```python
from build123d import *

# Parameters (mm, degrees)
BOSS_EXTRU_1_DEPTH      = 10
COQUE1_T                = 2.5
CONG_1_R                = 2
ESQUISSE3_R             = 3
ESQUISSE3_R_2           = 1.5
BOSS_EXTRU_2_DEPTH      = 9.43
ESQUISSE4_W             = 9.967172774
ESQUISSE4_H             = 2.559848265
ENL_V_MAT_EXTRU_2_DEPTH = 1
CONG_4_R                = 1
ESQUISSE5_R             = 1.7
ESQUISSE5_R_2           = 1.728785314
ESQUISSE5_R_3           = 14.25
ESQUISSE5_R_4           = 14.15
ENL_V_MAT_EXTRU_3_DEPTH = 10
ESQUISSE6_R             = 1.5
ENL_V_MAT_EXTRU_4_DEPTH = 10


# Some blends are built 0.0001 mm under size
with BuildPart() as part:
    # Esquisse1 → Boss.-Extru.1 (new body)
    with BuildSketch(Plane.XY):
        with BuildLine():
            Line((-34.96, -64), (34.96, -64))
            ThreePointArc((34.96, -64), (36.756051224, -63.256051224), (37.5, -61.46))
            Line((37.5, -61.46), (37.5, 61.46))
            ThreePointArc((37.5, 61.46), (36.756051224, 63.256051224), (34.96, 64))
            Line((34.96, 64), (-34.96, 64))
            ThreePointArc((-34.96, 64), (-36.756051224, 63.256051224), (-37.5, 61.46))
            Line((-37.5, 61.46), (-37.5, -61.46))
            ThreePointArc((-37.5, -61.46), (-36.756051224, -63.256051224), (-34.96, -64))
        make_face()
    extrude(amount=BOSS_EXTRU_1_DEPTH)

    # Coque1
    coque1_openings = [part.faces().sort_by_distance(p)[0] for p in [
        (0, 0, 10),
    ]]
    offset(amount=COQUE1_T, openings=coque1_openings, kind=Kind.INTERSECTION)

    # Congé1
    # the kernel refuses this fillet: 2 mm, written as the material it takes off along each edge
    with BuildSketch(Plane(origin=(34.96, 66.5, -2.5), x_dir=(0, 0, 1), z_dir=(-1, 0, 0)), Plane(origin=(-34.96, -66.5, -2.5), x_dir=(0, 0, 1), z_dir=(1, 0, 0))) as cong_1_piece_1:
        with BuildLine():
            CenterArc((CONG_1_R, -CONG_1_R), CONG_1_R, 90, 90)
            Line((0, -CONG_1_R), (0, 0))
            Line((0, 0), (CONG_1_R, 0))
        make_face()
    extrude(amount=69.92, mode=Mode.SUBTRACT)
    with BuildSketch(Plane(origin=(34.96, 61.46, -2.5), x_dir=(0, 1, 0), z_dir=(-1, 0, 0))) as cong_1_piece_2:
        with BuildLine():
            CenterArc((5.04 - CONG_1_R, -CONG_1_R), CONG_1_R, 0, 90)
            Line((5.04 - CONG_1_R, 0), (5.04, 0))
            Line((5.04, 0), (5.04, -CONG_1_R))
        make_face()
    revolve(axis=Axis((34.96, 61.46, -2.5), (0, 0, -1)), revolution_arc=90, mode=Mode.SUBTRACT)
    with BuildSketch(Plane(origin=(40, -61.46, -2.5), x_dir=(0, 0, 1), z_dir=(0, 1, 0)), Plane(origin=(-40, 61.46, -2.5), x_dir=(0, 0, 1), z_dir=(0, -1, 0))) as cong_1_piece_3:
        with BuildLine():
            CenterArc((CONG_1_R, -CONG_1_R), CONG_1_R, 90, 90)
            Line((0, -CONG_1_R), (0, 0))
            Line((0, 0), (CONG_1_R, 0))
        make_face()
    extrude(amount=122.92, mode=Mode.SUBTRACT)
    with BuildSketch(Plane(origin=(34.96, -61.46, -2.5), x_dir=(1, 0, 0), z_dir=(0, 1, 0))) as cong_1_piece_4:
        with BuildLine():
            CenterArc((5.04 - CONG_1_R, -CONG_1_R), CONG_1_R, 0, 90)
            Line((5.04 - CONG_1_R, 0), (5.04, 0))
            Line((5.04, 0), (5.04, -CONG_1_R))
        make_face()
    revolve(axis=Axis((34.96, -61.46, -2.5), (0, 0, -1)), revolution_arc=90, mode=Mode.SUBTRACT)
    with BuildSketch(Plane(origin=(-34.96, -61.46, -2.5), x_dir=(0, -1, 0), z_dir=(1, 0, 0))) as cong_1_piece_5:
        with BuildLine():
            CenterArc((5.04 - CONG_1_R, -CONG_1_R), CONG_1_R, 0, 90)
            Line((5.04 - CONG_1_R, 0), (5.04, 0))
            Line((5.04, 0), (5.04, -CONG_1_R))
        make_face()
    revolve(axis=Axis((-34.96, -61.46, -2.5), (0, 0, -1)), revolution_arc=90, mode=Mode.SUBTRACT)
    with BuildSketch(Plane(origin=(-34.96, 61.46, -2.5), x_dir=(-1, 0, 0), z_dir=(0, -1, 0))) as cong_1_piece_6:
        with BuildLine():
            CenterArc((5.04 - CONG_1_R, -CONG_1_R), CONG_1_R, 0, 90)
            Line((5.04 - CONG_1_R, 0), (5.04, 0))
            Line((5.04, 0), (5.04, -CONG_1_R))
        make_face()
    revolve(axis=Axis((-34.96, 61.46, -2.5), (0, 0, -1)), revolution_arc=90, mode=Mode.SUBTRACT)

    # Esquisse3 → Boss.-Extru.2 (add)
    # profile 1 of 4: a face of its own
    with BuildSketch(Plane.XY):
        with Locations(Location((-33.02, 59.69, 0), (0, 0, 180))):
            Circle(ESQUISSE3_R)
        with Locations(Location((-33.02, 59.69, 0), (0, 0, 180))):
            Circle(ESQUISSE3_R_2, mode=Mode.SUBTRACT)
    # profile 2 of 4: a face of its own
    with BuildSketch(Plane.XY):
        with Locations(Location((33.046544, 59.69, 0), (0, 0, 180))):
            Circle(ESQUISSE3_R)
        with Locations(Location((33.046544, 59.69, 0), (0, 0, 180))):
            Circle(ESQUISSE3_R_2, mode=Mode.SUBTRACT)
    # profile 3 of 4: a face of its own
    with BuildSketch(Plane.XY):
        with Locations(Location((-33.06, -59.69, 0), (0, 0, 180))):
            Circle(ESQUISSE3_R)
        with Locations(Location((-33.06, -59.69, 0), (0, 0, 180))):
            Circle(ESQUISSE3_R_2, mode=Mode.SUBTRACT)
    # profile 4 of 4: a face of its own
    with BuildSketch(Plane.XY):
        with Locations(Location((33.046483, -59.75896698, 0), (0, 0, 180))):
            Circle(ESQUISSE3_R)
        with Locations(Location((33.046483, -59.75896698, 0), (0, 0, 180))):
            Circle(ESQUISSE3_R_2, mode=Mode.SUBTRACT)
    extrude(amount=BOSS_EXTRU_2_DEPTH)

    # Esquisse4 → Enlèv. mat.-Extru.2 (cut)
    with BuildSketch(Plane.XY.offset(10)):
        with Locations((-24.5364, -65.279924132)):
            Rectangle(ESQUISSE4_W, ESQUISSE4_H)
    extrude(amount=-ENL_V_MAT_EXTRU_2_DEPTH, mode=Mode.SUBTRACT)

    # Congé4
    cong_4_edges = [part.edges().sort_by_distance(p)[0] for p in [
        (-19.552813613, -65.25, 9),
        (-29.519986387, -65.25, 9),
    ]]
    fillet(cong_4_edges, radius=CONG_4_R - 0.0001)  # a hair under: the kernel refuses the full size

    # Esquisse5 → Enlèv. mat.-Extru.3 (cut)
    with BuildSketch(Plane(origin=(0, 0, -2.5), x_dir=(-1, 0, 0), z_dir=(0, 0, -1))):
        with Locations((-13.048991778, 44.95809385)):
            Circle(ESQUISSE5_R)
        with Locations((10.751008222, 44.95809385)):
            Circle(ESQUISSE5_R)
        with Locations((10.751008222, 21.15809385)):
            Circle(ESQUISSE5_R)
        with Locations((-13.048991778, 21.15809385)):
            Circle(ESQUISSE5_R)
        with Locations((-13.048991778, 9.795871187)):
            Circle(ESQUISSE5_R_2)
        with Locations((10.751008222, 9.824656501)):
            Circle(ESQUISSE5_R)
        with Locations((10.751008222, -13.975343499)):
            Circle(ESQUISSE5_R)
        with Locations((-13.048991778, -13.975343499)):
            Circle(ESQUISSE5_R)
        with Locations((-13.048991778, -25.396338685)):
            Circle(ESQUISSE5_R)
        with Locations((10.751008222, -25.396338685)):
            Circle(ESQUISSE5_R)
        with Locations((10.751008222, -49.196338685)):
            Circle(ESQUISSE5_R)
        with Locations((-13.048991778, -49.196338685)):
            Circle(ESQUISSE5_R)
        with Locations((-1.148991778, -37.296338685)):
            Circle(ESQUISSE5_R_3)
        with Locations((-1.148991778, -2.075343499)):
            Circle(ESQUISSE5_R_3)
        with Locations((-1.148991778, 33.05809385)):
            Circle(ESQUISSE5_R_4)
    extrude(amount=-ENL_V_MAT_EXTRU_3_DEPTH, mode=Mode.SUBTRACT)

    # Esquisse6 → Enlèv. mat.-Extru.4 (cut)
    with BuildSketch(Plane.XY):
        with Locations((25.740105724, 16.653070924)):
            Circle(ESQUISSE6_R)
        with Locations((25.740105724, -19.683006416)):
            Circle(ESQUISSE6_R)
        with Locations((25.740105724, -54.120805544)):
            Circle(ESQUISSE6_R)
    extrude(amount=-ENL_V_MAT_EXTRU_4_DEPTH, mode=Mode.SUBTRACT)


solid = part.part
```
Source: CAD feature listing. Evaluate the final solid. Frame: model axes, mm. A direction names the side the tool comes from. Give positions to 0.01 mm unless a question says otherwise; leave off trailing zeros. Loops run counter-clockwise (first coordinate to the right, second up) from the corner with the lowest first, then second, coordinate; pieces in that order, holes last. Notation, with made-up numbers: (74.5, 78.25) -> (131.5, 78.25) arc R9 cw to (131.5, 90.25) -> close; hole circle Ø9 at (53.5, 37.25). An arc over 180 degrees is marked (long way). Put each result on its own line as item: value. Start each with the question number.
1) Cut plane D-D (y = 59.69). Return loops of the section in (x, z), then the cut area to 3 significant figures.
2) Cut plane A-A (z = 4.75). State how many separate pieces and enclosed holes the cut face has, then the cut area to 3 significant figures.
3) Contact query for flat-ended pins moving along their axis: P1, Ø5, axis at x = -32, y = -60, coming from the +Z side; P2, Ø5.5, axis at x = 13.05, y = 9.8, coming from the +Z side. Output: stop coordinate, or through.
4) Cut plane B-B (y = 28). Return loops of the section in (x, z).
5) Reachability of faces 1 (the face through (12.457, -10.746, -1.268)), 2 (the face through (33.242, -61.246, 4.649)) from +Z, -Z, +X, -X, +Y, -Y: full face, straight path, thin tool, end or side. Return the list, or none.
6) Cut plane C-C (x = 7.5). Return loops of the section in (y, z), then the cut area to 3 significant figures.
7) Draft query along Y for faces 3 (the face through (-25, -65, 9)), 4 (the face through (38.563, 64.984, 4.676)), 5 (the face through (33, 60, 0)). Return one class per face: released by +Y, released by -Y, zero draft, split by the parting line, or undercut.
8) Material intervals for probe 1 along Y at (x, z) = (-33.02, 4.75); probe 2 along Y at (x, z) = (-25, 1); probe 3 along X at (y, z) = (23.5, 8), sorted ascending.
Results are:
1. outline: (-40, -0.5) arc R2 ccw to (-38, -2.5) -> (38, -2.5) arc R2 ccw to (40, -0.5) -> (40, 10) -> (37.5, 10) -> (37.5, 0) -> (36.05, 0) -> (36.05, 9.43) -> (34.55, 9.43) -> (34.55, 0) -> (31.55, 0) -> (31.55, 9.43) -> (30.05, 9.43) -> (30.05, 0) -> (-30.02, 0) -> (-30.02, 9.43) -> (-31.52, 9.43) -> (-31.52, 0) -> (-34.52, 0) -> (-34.52, 9.43) -> (-36.02, 9.43) -> (-36.02, 0) -> (-37.5, 0) -> (-37.5, 10) -> (-40, 10) -> close
1. area: 305 mm2
2. separate pieces: 5
2. enclosed holes: 5
2. area: 1,110 mm2
3. P1: stops at z = 9.43
3. P2: stops at z = 0
4. outline: (-40, -0.5) arc R2 ccw to (-38, -2.5) -> (-12.07, -2.5) -> (-12.07, 0) -> (-37.5, 0) -> (-37.5, 10) -> (-40, 10) -> close; (14.36, -2.5) -> (38, -2.5) arc R2 ccw to (40, -0.5) -> (40, 10) -> (37.5, 10) -> (37.5, 0) -> (14.36, 0) -> close
5. face 1: +Z, -Z
5. face 2: +Z
6. outline: (-66.5, -0.5) arc R2 ccw to (-64.5, -2.5) -> (-50.05, -2.5) -> (-50.05, 0) -> (-64, 0) -> (-64, 10) -> (-66.5, 10) -> close; (-24.54, -2.5) -> (-14.83, -2.5) -> (-14.83, 0) -> (-24.54, 0) -> close; (10.68, -2.5) -> (20.41, -2.5) -> (20.41, 0) -> (10.68, 0) -> close; (45.7, -2.5) -> (64.5, -2.5) arc R2 ccw to (66.5, -0.5) -> (66.5, 10) -> (64, 10) -> (64, 0) -> (45.7, 0) -> close
6. area: 190 mm2
7. face 3: zero draft
7. face 4: released by +Y
7. face 5: undercut
8. probe 1: y = -66.5 to -64, -62.69 to -61.19, -58.19 to -56.69, 56.69 to 58.19, 61.19 to 62.69, 64 to 66.5
8. probe 2: y = -66.5 to -64, 64 to 66.5
8. probe 3: x = -40 to -37.5, 37.5 to 40
